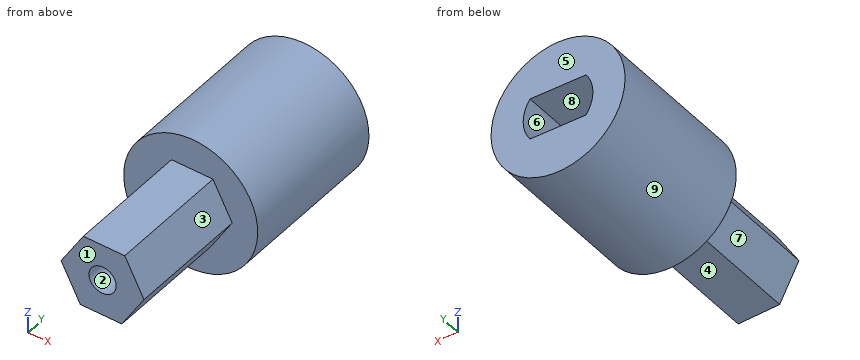
from build123d import *

# Parameters (mm, degrees)
SALIENTE_EXTRUIR1_DEPTH = 11.5
CROQUIS2_R              = 6.15
SALIENTE_EXTRUIR2_DEPTH = 14.51
CROQUIS3_R              = 1.25
CORTAR_EXTRUIR1_DEPTH   = 8
CORTAR_EXTRUIR2_DEPTH   = 8


with BuildPart() as part:
    # Croquis1 → Saliente-Extruir1 (new body)
    with BuildSketch(Plane(origin=(0, 0, 0), x_dir=(1, 0, 0), z_dir=(0, 1, 0))):
        Polygon((2.041290993, -3.217628176), (3.807193237, 0.158995769), (1.765902244, 3.376623945), (-2.041290993, 3.217628176), (-3.807193237, -0.158995769), (-1.765902244, -3.376623945), align=None)
    extrude(amount=SALIENTE_EXTRUIR1_DEPTH)

    # Croquis2 → Saliente-Extruir2 (add)
    with BuildSketch(Plane(origin=(0, 11.5, 0), x_dir=(1, 0, 0), z_dir=(0, 1, 0))):
        with Locations(Location((0, 0, 0), (0, 0, 270))):
            Circle(CROQUIS2_R)
    extrude(amount=SALIENTE_EXTRUIR2_DEPTH)

    # Croquis3 → Cortar-Extruir1 (cut)
    with BuildSketch(Plane.XZ):
        with Locations(Location((0, 0, 0), (0, 0, 270))):
            Circle(CROQUIS3_R)
    extrude(amount=-CORTAR_EXTRUIR1_DEPTH, mode=Mode.SUBTRACT)

    # Croquis4 → Cortar-Extruir2 (cut)
    with BuildSketch(Plane(origin=(0, 26.01, 0), x_dir=(1, 0, 0), z_dir=(0, 1, 0))):
        with BuildLine():
            Line((-2.574878638, 1.9), (2.574878638, 1.9))
            ThreePointArc((2.574878638, 1.9), (3.2, 0), (2.574878638, -1.9))
            Line((2.574878638, -1.9), (-2.574878638, -1.9))
            ThreePointArc((-2.574878638, -1.9), (-3.2, 0), (-2.574878638, 1.9))
        make_face()
    extrude(amount=-CORTAR_EXTRUIR2_DEPTH, mode=Mode.SUBTRACT)


solid = part.part
CAD build for the part. Positions are in the model's coordinates, mm. Face numbers are marked on the shaded views. A direction names the side the tool comes from. Coordinates: 2 decimals unless noted, no trailing zeros. Loops run counter-clockwise (first coordinate to the right, second up) from the corner with the lowest first, then second, coordinate; pieces in that order, holes last. Notation, with made-up numbers: (-27.5, 51) - (-15.5, 51) arc R22 cw to (-15.5, 74) - close; hole circle Ø3 at (83, 62.25). An arc over 180 degrees is marked (long way). Write item = value, one per line. Start each with the question number.
Q1. Cut at D-D, the plane y = 12.5. List the corners of the cut face in (x, z), then the cut area to 3 significant figures.
Q2. Drill centre lines: L1, parallel to Y at x = -3, z = -2.75; L2, parallel to Z at x = -0.25, y = 21.75; L3, parallel to X at y = 2, z = 0. Where is each one in solid material? Low to high.
Q3. Flat gauge pins, fed straight in: pin 1 Ø3 at (x, z) = (0.5, 0) entering from +Y; pin 2 Ø1.5 at (x, z) = (4.5, -2) entering from -Y; pin 3 Ø6 at (x, y) = (-4, 6) entering from +Z. Where does each tip first touch, or does it go through?
Q4. Cut at A-A, the plane y = 7. List the corners of the cut face in (x, z).
Q5. Cut at C-C, the plane z = -2.25. List the corners of the cut face in (x, y).
Q6. Pull direction X, two halves, no side cores. Call the marked faces 6, 7, 8 and 9: pulls with the +X half, pulls with the -X half, needs draft (parallel to the pull), parting line crosses it, or undercut.
Q7. Which spindle directions (+Z, -Z, +X, -X, +Y, -Y) get a long thin tool onto all of the face, cutting with end or side? Do the marked faces 1, 2, 3, 4 and 5. Say none if no direction does.
Q8. Cut at B-B, the plane x = 3.5. List the corners of the cut face in (y, z).
Computed:
q1.outline = circle Ø12.3 at (0, 0)
q1.area = 119 mm²
q2.L1 = 11.5 to 26.01
q2.L2 = -6.14 to -1.9, 1.9 to 6.14
q2.L3 = -3.72 to -1.25, 1.25 to 3.72
q3.pin_1 = 18.01
q3.pin_2 = 11.5
q3.pin_3 = 3.38
q4.outline = (-3.81, 0.16) - (-2.04, -3.22) - (1.77, -3.38) - (3.81, -0.16) - (2.04, 3.22) - (-1.77, 3.38) - close; hole circle Ø2.5 at (0, 0)
q5.outline = (-5.72, 11.5) - (-2.55, 11.5) - (-2.55, 0) - (2.48, 0) - (2.48, 11.5) - (5.72, 11.5) - (5.72, 26.01) - (-5.72, 26.01) - close
q6.face_6 = undercut
q6.face_7 = pulls with the -X half
q6.face_8 = undercut
q6.face_9 = parting line crosses it
q7.face_1 = +Z, -Z, +X, -X, -Y
q7.face_2 = -Y
q7.face_3 = +Z, +X, -Y
q7.face_4 = -Z, -X, -Y
q7.face_5 = +Z, -Z, +X, -X, +Y
q8.outline = (0, -0.64) - (11.5, -0.64) - (11.5, -5.06) - (26.01, -5.06) - (26.01, 5.06) - (11.5, 5.06) - (11.5, 0.43) - (0, 0.43) - close
